The model under review builds one solid part; all positions refer to its coordinate system, in mm. A direction names the side the tool comes from. Give positions to 0.01 mm unless a question says otherwise; leave off trailing zeros. Order: outer loops, then holes, each group sorted by start corner. A loop starts at its lowest first (then second) coordinate and runs counter-clockwise, first axis right, second up.
```python
from build123d import *

# Parameters (mm, degrees)
F0_R     = 10
F1_DEPTH = 12.5
F2_R     = 12.5
F2_R_2   = 7.5
F3_DEPTH = 3
F4_R     = 10
F4_R_2   = 7.5
F5_DEPTH = 10


with BuildPart() as f1:
    # F0 (on Front) → F1 (new body)
    with BuildSketch(Plane.XZ):
        with BuildLine():
            Line((6.25, 15), (-6.25, 15))
            ThreePointArc((-6.25, 15), (-8.125, 14.072913), (-9.865381, 12.912659))
            Line((-9.865381, 12.912659), (-16.115381, 2.087341))
            ThreePointArc((-16.115381, 2.087341), (-16.25, 0), (-16.115381, -2.087341))
            Line((-16.115381, -2.087341), (-9.865381, -12.912659))
            ThreePointArc((-9.865381, -12.912659), (-8.125, -14.072913), (-6.25, -15))
            Line((-6.25, -15), (6.25, -15))
            ThreePointArc((6.25, -15), (8.125, -14.072913), (9.865381, -12.912659))
            Line((9.865381, -12.912659), (16.115381, -2.087341))
            ThreePointArc((16.115381, -2.087341), (16.21631, -1.045839), (16.25, 0))
            ThreePointArc((16.25, 0), (16.21631, 1.045839), (16.115381, 2.087341))
            Line((16.115381, 2.087341), (9.865381, 12.912659))
            ThreePointArc((9.865381, 12.912659), (8.125, 14.072913), (6.25, 15))
        make_face()
        Circle(F0_R, mode=Mode.SUBTRACT)
    extrude(amount=F1_DEPTH)

    # F2 (on face) → F3 (join)
    with BuildSketch(Plane.XZ.offset(12.5)):
        Circle(F2_R)
        Circle(F2_R_2, mode=Mode.SUBTRACT)
    extrude(amount=F3_DEPTH)

    # F4 (on face) → F5 (join)
    with BuildSketch(Plane.XZ.offset(15.5)):
        Circle(F4_R)
        Circle(F4_R_2, mode=Mode.SUBTRACT)
    extrude(amount=F5_DEPTH)


solid = f1.part
```
Item 1: Take a section at A-A (x = 0). Give the boundary of the cut face in (y, z), and give its area (3 significant figures).
Values found:
outline: (-25.5, -10) - (-15.5, -10) - (-15.5, -12.5) - (-12.5, -12.5) - (-12.5, -15) - (0, -15) - (0, -10) - (-12.5, -10) - (-12.5, -7.5) - (-25.5, -7.5) - close; (-25.5, 7.5) - (-12.5, 7.5) - (-12.5, 10) - (0, 10) - (0, 15) - (-12.5, 15) - (-12.5, 12.5) - (-15.5, 12.5) - (-15.5, 10) - (-25.5, 10) - close
area: 205 mm2
Item 2: For line 1 (Z direction, x = 0, y = -16.5); line 2 (Z direction, x = 0, y = -9.25); line 3 (Y direction, x = -8.5, z = 3), list the stretches that pass through material, from the lowest coordinate up.
Values found:
line 1: z = -10 to -7.5, 7.5 to 10
line 2: z = -15 to -10, 10 to 15
line 3: y = -25.5 to -12.5
Item 3: Take a section at D-D (z = -4). Give the boundary of the cut face in (x, y).
Values found:
outline: (-15.01, -12.5) - (-11.84, -12.5) - (-11.84, -15.5) - (-9.17, -15.5) - (-9.17, -25.5) - (-6.34, -25.5) - (-6.34, -12.5) - (-9.17, -12.5) - (-9.17, 0) - (-15.01, 0) - close; (6.34, -25.5) - (9.17, -25.5) - (9.17, -15.5) - (11.84, -15.5) - (11.84, -12.5) - (15.01, -12.5) - (15.01, 0) - (9.17, 0) - (9.17, -12.5) - (6.34, -12.5) - close
Item 4: Take a section at C-C (z = -12). Give the boundary of the cut face in (x, y).
Values found:
outline: (-10.39, -12.5) - (-3.5, -12.5) - (-3.5, -15.5) - (3.5, -15.5) - (3.5, -12.5) - (10.39, -12.5) - (10.39, 0) - (-10.39, 0) - close
Item 5: Draft analysis for pull direction Z (two halves, no side actions). For faces 3 (the cylindrical face through (-8.15, -6.16, -14.06)), 4 (the flat face through (4, -25.5, 7)), 5 (the cylindrical face through (-2.17, -6.16, -9.76)), state which applies: released by +Z, released by -Z, zero draft, split by the parting line, or undercut.
Values found:
face 3: released by -Z
face 4: zero draft
face 5: undercut
Item 6: Take a section at B-B (y = -10). Give the boundary of the cut face in (x, z).
Values found:
outline: (-16.12, -2.09) - (-9.87, -12.91) arc R16.25 ccw to (-6.25, -15) - (6.25, -15) arc R16.25 ccw to (9.87, -12.91) - (16.12, -2.09) arc R16.25 ccw to (16.25, 0) arc R16.25 ccw to (16.12, 2.09) - (9.87, 12.91) arc R16.25 ccw to (6.25, 15) - (-6.25, 15) arc R16.25 ccw to (-9.87, 12.91) - (-16.12, 2.09) arc R16.25 ccw to start; hole circle Ø20 at (0, 0)
Item 7: For faces 1 (the cylindrical face through (-7.493, -18.909, 0.33)), 2 (the flat face through (-0.1, -15.5, 10.2)), list the 3-axis set-ups (+Z, -Z, +X, -X, +Y, -Y) from which the entire face can be reached by the end or side of a thin tool; tool diameter is ignored.
Values found:
face 1: +Y, -Y
face 2: -Y
Item 8: Clearance check with flat-ended pins moving along their axes: pin 1 Ø7.5 at (x, z) = (-5.5, -1) entering from -Y; pin 2 Ø12 at (x, z) = (0, 0) entering from +Y; pin 3 Ø5 at (x, y) = (1.5, -18.5) entering from -Z; pin 4 Ø1 at (y, z) = (-14, 1) entering from -X. State where each tip first meets the part, or that it passes through.
Values found:
pin 1: stops at y = -25.5
pin 2: passes through
pin 3: stops at z = -10
pin 4: stops at x = -12.49
